from build123d import *

# Parameters (mm, degrees)
SKETCH1_W           = 15
SKETCH1_H           = 10
BOSS_EXTRUDE1_DEPTH = 1.5
BOSS_EXTRUDE2_DEPTH = 4
SKETCH3_W           = 2.5
SKETCH3_H           = 10
CUT_EXTRUDE1_DEPTH  = 1.5


with BuildPart() as part:
    # Sketch1 → Boss-Extrude1 (new body)
    with BuildSketch(Plane(origin=(0, 0, 0), x_dir=(1, 0, 0), z_dir=(0, 1, 0))):
        Rectangle(SKETCH1_W, SKETCH1_H)
    extrude(amount=BOSS_EXTRUDE1_DEPTH)

    # Sketch2 → Boss-Extrude2 (add)
    with BuildSketch(Plane(origin=(0, 1.5, 0), x_dir=(1, 0, 0), z_dir=(0, 1, 0))):
        with BuildLine():
            Line((-6, 3.4), (0, 3.4))
            ThreePointArc((0, 3.4), (2.9, 0.5), (0, -2.4))
            Line((0, -2.4), (-6, -2.4))
            ThreePointArc((-6, -2.4), (-6.778585026, -2.293529194), (-7.5, -1.981934729))
            Line((-7.5, -1.981934729), (-7.5, 2.981934729))
            ThreePointArc((-7.5, 2.981934729), (-6.778585026, 3.293529194), (-6, 3.4))
        make_face()
    extrude(amount=BOSS_EXTRUDE2_DEPTH)

    # Sketch3 → Cut-Extrude1 (cut)
    with BuildSketch(Plane.XZ):
        with Locations((-0.5, 0)):
            Rectangle(SKETCH3_W, SKETCH3_H)
    extrude(amount=-CUT_EXTRUDE1_DEPTH, mode=Mode.SUBTRACT)


solid = part.part
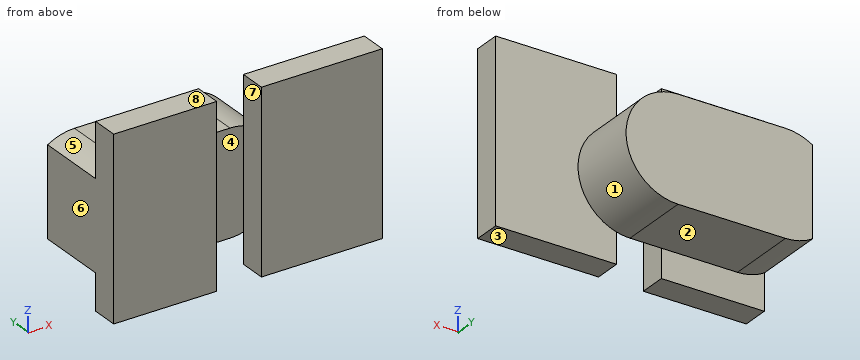
Could you check a few things on this model? Use its own coordinates, in mm. Face numbers are marked on the shaded views. A direction names the side the tool comes from. Give positions to 0.01 mm unless a question says otherwise; leave off trailing zeros. Order: outer loops, then holes, each group sorted by start corner. A loop starts at its lowest first (then second) coordinate and runs counter-clockwise, first axis right, second up. Notation, with made-up numbers: (24.25, 32) - (33.25, 32) arc R24 ccw to (33.25, 48) - close; hole circle Ø11 at (32.5, -23). An arc over 180 degrees is marked (long way). Return JSON: item names as keys, results as strings. Group by question number.
Q1. Suppose I cut it at D-D, the plane z = -0.5. Please give me the cut outline in (x, y), and give its area (4 significant figures).
Q2. Please list where these lines run through material, in increasing order: line 1 along X through (y, z) = (0.65, 1.5); line 2 along Y through (x, z) = (-6, 4); line 3 along Z through (x, y) = (-4.25, 3.7). Write a range as [from, to].
Q3. Which directions (+Z, -Z, +X, -X, +Y, -Y) give clear straight access to the entire face, cutting with the end or side of a thin tool? Please do the marked faces 1, 2, 3, 4 and 5.
Q4. Thinking about a two-plate mould opening in X: for the marked faces 6, 7 and 8, which applies, pulls with the +X half, pulls with the -X half, needs draft (parallel to the pull), parting line crosses it, or undercut?
Q5. Suppose I cut it at C-C, the plane y = 3.1. Please give me the cut outline in (x, z), and give its area (3 significant figures).
Q6. Will these pins go through, and if not, where does the flat tip stop? pin 1 Ø2 at (x, y) = (-6, 4.5) entering from +Z; pin 2 Ø0.6 at (x, z) = (-6, -4.5) entering from +Y; pin 3 Ø3 at (x, y) = (-3, 3.5) entering from -Z; pin 4 Ø3 at (x, z) = (-1, -1.5) entering from -Y.
Q7. Suppose I cut it at A-A, the plane z = -3.75. Please give me the cut outline in (x, y), and give its area (4 significant figures).
Q8. Suppose I cut it at B-B, the plane x = -4. Please give me the cut outline in (y, z), and give its area (3 significant figures).
Resolved:
{
 "1": {"outline": "(-7.5, 0) - (-1.75, 0) - (-1.75, 1.5) - (0.75, 1.5) - (0.75, 0) - (7.5, 0) - (7.5, 1.5) - (2.9, 1.5) - (2.9, 5.5) - (-7.5, 5.5) - close", "area": "60.35 mm2"},
 "2": {"line 1": "x = [-7.5, -1.75], [0.75, 7.5]", "line 2": "y = [0, 1.5]", "line 3": "z = [-3.4, 2.4]"},
 "3": {"face 1": "+X, +Y", "face 2": "-Z, +X, -X, +Y", "face 3": "-Z, +X, -X, +Y, -Y", "face 4": "+Z, -Z, -Y", "face 5": "+Z, -X, +Y"},
 "4": {"face 6": "pulls with the -X half", "face 7": "undercut", "face 8": "needs draft"},
 "5": {"outline": "(-7.5, -2.98) arc R2.9 ccw to (-6, -3.4) - (0, -3.4) arc R2.9 ccw to (0, 2.4) - (-6, 2.4) arc R2.9 ccw to (-7.5, 1.98) - close", "area": "56.3 mm2"},
 "6": {"pin 1": "stops at z = 2.4", "pin 2": "stops at y = 1.5", "pin 3": "stops at z = -3.4", "pin 4": "stops at y = 0"},
 "7": {"outline": "(-7.5, 0) - (-1.75, 0) - (-1.75, 1.5) - (-7.5, 1.5) - close; (0.75, 0) - (7.5, 0) - (7.5, 1.5) - (0.75, 1.5) - close", "area": "18.75 mm2"},
 "8": {"outline": "(0, -5) - (1.5, -5) - (1.5, -3.4) - (5.5, -3.4) - (5.5, 2.4) - (1.5, 2.4) - (1.5, 5) - (0, 5) - close", "area": "38.2 mm2"}
}
